```python
from build123d import *

# Parameters (mm, degrees)
F0_R     = 2
F1_DEPTH = 2


with BuildPart() as f1:
    # F0 (on Top) → F1 (new body)
    with BuildSketch(Plane.XY):
        Polygon((26.7, 20.675), (26.7, 34.175), (-26.7, 34.175), (-26.7, 21.675), (-26.7, -34.175), (-19.95, -34.175), (8.45, -34.175), (26.7, -34.175), align=None)
        with BuildLine():
            ThreePointArc((-17.95, -31.425), (-18.535786, -32.839214), (-19.95, -33.425))
            ThreePointArc((-19.95, -33.425), (-21.364214, -30.010786), (-17.95, -31.425))
        make_face(mode=Mode.SUBTRACT)
        with BuildLine():
            ThreePointArc((10.45, -31.175), (9.864214, -32.589214), (8.45, -33.175))
            ThreePointArc((8.45, -33.175), (7.035786, -29.760786), (10.45, -31.175))
        make_face(mode=Mode.SUBTRACT)
        with BuildLine():
            ThreePointArc((-21.95, 21.675), (-23.95, 19.675), (-25.95, 21.675))
            ThreePointArc((-25.95, 21.675), (-23.95, 23.675), (-21.95, 21.675))
        make_face(mode=Mode.SUBTRACT)
        with Locations((23.7, 20.675)):
            Circle(F0_R, mode=Mode.SUBTRACT)
    extrude(amount=F1_DEPTH)


solid = f1.part
```
Check sheet for the modelled part. Datum: model origin and axes. Units: mm. Round coordinates to 2 decimals unless told otherwise and drop trailing zeros. Loops run counter-clockwise (first coordinate to the right, second up) from the corner with the lowest first, then second, coordinate; pieces in that order, holes last. Notation, with made-up numbers: (8.5, 4.25) -> (56.5, 4.25) arc R7 cw to (56.5, 12.25) -> close; hole circle Ø11 at (76, 89). An arc over 180 degrees is marked (long way). Write item = value, one per line. Start each with the question number.
1) Sectioned sample at A-A, the plane x = 23.7. Record the cut outline in (y, z) (3 decimals).
2) Gauge pin test, flat end, axial feed: pin 1 Ø3.5 at (x, y) = (-19.95, -31.425) entering from -Z. Record the tip position at first contact, or that the pin passes through.
3) Release check for a two-part mould opening along Y. For faces 1 (the flat face through (0, 0, 2)), 2 (the cylindrical face through (24.78, 22.36, 0.99)), 3 (the flat face through (0, -34.175, 1)), 4 (the cylindrical face through (-25.03, 23.36, 0.99)) record: released by +Y, released by -Y, zero draft, split by the parting line, or undercut.
4) Thickness scan on probe 1 along Y at (x, z) = (-19.95, 0.5) (3 decimals); probe 2 along Y at (x, z) = (23.7, 1.25) (3 decimals). Record the ranges inside material, lowest first.
Results are:
q1.outline = (-34.175, 0) -> (18.675, 0) -> (18.675, 2) -> (-34.175, 2) -> close; (22.675, 0) -> (34.175, 0) -> (34.175, 2) -> (22.675, 2) -> close
q2.pin_1 = through
q3.face_1 = zero draft
q3.face_2 = undercut
q3.face_3 = released by -Y
q3.face_4 = undercut
q4.probe_1 = -34.175 to -33.425, -29.425 to 34.175
q4.probe_2 = -34.175 to 18.675, 22.675 to 34.175
